Verification items for the finished model (mm, model axes). Face numbers are marked on the shaded views. A direction names the side the tool comes from. Round coordinates to 2 decimals unless told otherwise and drop trailing zeros. Order: outer loops, then holes, each group sorted by start corner. A loop starts at its lowest first (then second) coordinate and runs counter-clockwise, first axis right, second up. Notation, with made-up numbers: M 88.5,53 L 93.5,53 A33 ccw 93.5,84 Z; hole C -37.75,-11.75 d3. An arc over 180 degrees is marked long. Use one line per item in the form item = value. Start each with the question number.
Item 1: Tool access check on the marked faces 1 and 2. Record the directions out of +Z, -Z, +X, -X, +Y, -Y that give a thin tool (end or side, any length) a straight path to the whole face; none if there is none.
Item 2: Thickness scan on probe 1 along Z at (x, y) = (6, -30); probe 2 along Y at (x, z) = (9.5, 28.5); probe 3 along Y at (x, z) = (11.5, 51). Record the ranges inside material, lowest first. Write a range as [from, to].
Item 3: Go/stop test with flat-tipped pins: pin 1 Ø10 at (x, z) = (23, 29.5) entering from -Y; pin 2 Ø10 at (x, z) = (-20.5, 25) entering from +Y; pin 3 Ø5 at (x, z) = (-24, 16.5) entering from +Y. Record where each tip stops, or that it passes through.
Item 4: Cross-section at B-B on y = -24. Enter the section's corners in (x, z).
Item 5: Cross-section at A-A on y = 26.5. Count the separate pieces of the cut face and the enclosed holes in it, then the cut area to 3 significant figures.
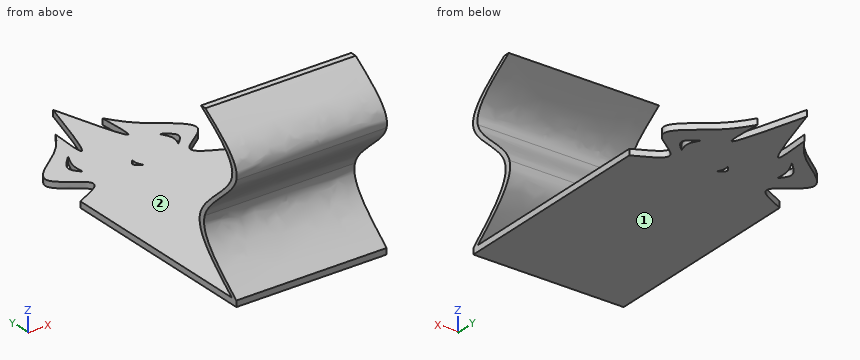
from build123d import *

# Parameters (mm, degrees)
F1_DEPTH = 2.54
F3_DEPTH = 63.5


with BuildPart() as f1:
    # F0 (on Top) → F1 (new body)
    with BuildSketch(Plane.XY):
        with BuildLine():
            Line((-31.75, -83.6839513757), (31.75, -83.6839513778))
            Line((31.75, -83.6839513778), (31.75, 5.2160486222))
            add(Edge.make_bspline(
                [(31.75, 5.2160486243), (25.7086750977, 8.2095040737), (13.2919018227, 13.2612920956), (40.4686708732, 24.151033206), (17.1693446816, 37.3717586227), (12.2441961548, 45.1813499568), (9.8845292789, 48.7718827984)],
                knots=[0, 0, 0, 0, 0.2366640156, 0.4851512444, 0.756842013, 1, 1, 1, 1], degree=3))
            add(Edge.make_bspline(
                [(9.8845292789, 48.7718827984), (10.3444855628, 41.5162894514), (11.4748144078, 23.6858829352), (4.2718916672, 48.7681543781), (0, 63.6438973943)],
                knots=[0, 0, 0, 0, 0.4069224168, 1, 1, 1, 1], degree=3))
            add(Edge.make_bspline(
                [(-9.8845292789, 48.7718827984), (-10.3444855628, 41.5162894514), (-11.4748144078, 23.6858829352), (-4.2718916672, 48.7681543781), (0, 63.6438973943)],
                knots=[0, 0, 0, 0, 0.4069224168, 1, 1, 1, 1], degree=3))
            add(Edge.make_bspline(
                [(-31.75, 5.2160486243), (-25.7086750977, 8.2095040737), (-13.2919018227, 13.2612920956), (-40.4686708732, 24.151033206), (-17.1693446816, 37.3717586227), (-12.2441961548, 45.1813499568), (-9.8845292789, 48.7718827984)],
                knots=[0, 0, 0, 0, 0.2366640156, 0.4851512444, 0.756842013, 1, 1, 1, 1], degree=3))
            Line((-31.75, 5.2160486243), (-31.75, -83.6839513757))
        make_face()
        with BuildLine():
            add(Edge.make_bspline(
                [(0, 18.4377846975), (-0.8402767268, 17.5937250168), (-2.6308980883, 15.7950420042), (-0.1427417595, 14.228570259), (1.1778091829, 13.3971894932)],
                knots=[0, 0, 0, 0, 0.4692654392, 1, 1, 1, 1], degree=3))
            add(Edge.make_bspline(
                [(0, 18.4377846975), (-0.0824907332, 17.6625700732), (-0.2575054179, 16.0178521281), (0.6814285359, 14.3035037553), (1.1778091829, 13.3971894932)],
                knots=[0, 0, 0, 0, 0.471335989, 1, 1, 1, 1], degree=3))
        make_face(mode=Mode.SUBTRACT)
        with BuildLine():
            add(Edge.make_bspline(
                [(-15.9456048132, 33.5736688751), (-16.9306722249, 31.6219338837), (-18.8522437067, 27.8146830449), (-18.5188141617, 23.8680684012), (-18.3563127499, 21.9446315956)],
                knots=[0, 0, 0, 0, 0.5126363558, 1, 1, 1, 1], degree=3))
            add(Edge.make_bspline(
                [(-18.3563127499, 21.9446315956), (-19.7054262057, 23.386298555), (-22.7926148104, 26.6852777417), (-18.411919139, 31.0924491189), (-15.9456048132, 33.5736688751)],
                knots=[0, 0, 0, 0, 0.4370039013, 1, 1, 1, 1], degree=3))
        make_face(mode=Mode.SUBTRACT)
        with BuildLine():
            add(Edge.make_bspline(
                [(18.4678306852, 28.4819673923), (19.427421291, 26.8806889301), (21.1201724035, 24.0559786368), (20.4629903584, 20.881000871), (19.9780060806, 19.4686195152), (19.7560574985, 18.8222556485)],
                knots=[0, 0, 0, 0, 0.4151573771, 0.7323521239, 1, 1, 1, 1], degree=3))
            add(Edge.make_bspline(
                [(18.4678306852, 28.4819673923), (20.8235774768, 26.9635696387), (25.4215767631, 23.9999267161), (21.6132297579, 20.51951007), (19.7560574985, 18.8222556485)],
                knots=[0, 0, 0, 0, 0.5123416723, 1, 1, 1, 1], degree=3))
        make_face(mode=Mode.SUBTRACT)
    extrude(amount=F1_DEPTH)

    # F2 (on face) → F3 (join)
    with BuildSketch(Plane.YZ.offset(31.75)):
        with BuildLine():
            add(Edge.make_bspline(
                [(-65.6484358175, 27.4432951095), (-67.9772508721, 34.9822299474), (-81.8557368461, 41.970962749), (-83.6839513778, 48.8775275409)],
                knots=[0.3464011194, 0.3464011194, 0.3464011194, 0.3464011194, 0.6770339361, 0.6770339361, 0.6770339361, 0.6770339361], degree=3))
            Line((-65.6484358175, 27.4432951095), (-63.1084358175, 27.4432951095))
            add(Edge.make_bspline(
                [(-81.1439513778, 48.8775275409), (-79.3157352707, 41.9709626757), (-65.4372513089, 34.9822301927), (-63.1084358175, 27.4432951095)],
                knots=[0.3229660639, 0.3229660639, 0.3229660639, 0.3229660639, 0.6535988806, 0.6535988806, 0.6535988806, 0.6535988806], degree=3))
            Line((-81.1439513778, 48.8775275409), (-83.6839513778, 48.8775275409))
        make_face()
        with BuildLine():
            add(Edge.make_bspline(
                [(-83.6839513778, 48.8775275409), (-85.4697730551, 55.6239420932), (-75.7576902273, 62.2919550981), (-66.0456140927, 68.9599682055)],
                knots=[0.6770339361, 0.6770339361, 0.6770339361, 0.6770339361, 1, 1, 1, 1], degree=3))
            Line((-83.6839513778, 48.8775275409), (-81.1439513778, 48.8775275409))
            add(Edge.make_bspline(
                [(-63.5056140927, 68.9599682055), (-73.2176967282, 62.2919556151), (-82.929774594, 55.6239421648), (-81.1439513778, 48.8775275409)],
                knots=[0, 0, 0, 0, 0.3229660639, 0.3229660639, 0.3229660639, 0.3229660639], degree=3))
            Line((-63.5056140927, 68.9599682055), (-66.0456140927, 68.9599682055))
        make_face()
        with BuildLine():
            add(Edge.make_bspline(
                [(-83.6839513778, 2.54), (-73.4462547351, 11.0424093805), (-63.2085565888, 19.5448188091), (-65.6484358175, 27.4432951095)],
                knots=[0, 0, 0, 0, 0.3464011194, 0.3464011194, 0.3464011194, 0.3464011194], degree=3))
            Line((-83.6839513778, 2.54), (-81.1439513778, 2.54))
            add(Edge.make_bspline(
                [(-63.1084358175, 27.4432951095), (-60.6685561312, 19.5448185522), (-70.9062511318, 11.0424082477), (-81.1439513778, 2.54)],
                knots=[0.6535988806, 0.6535988806, 0.6535988806, 0.6535988806, 1, 1, 1, 1], degree=3))
            Line((-63.1084358175, 27.4432951095), (-65.6484358175, 27.4432951095))
        make_face()
    extrude(amount=-F3_DEPTH)


solid = f1.part
Output values:
q1.face_1 = -Z, +X, -X, +Y, -Y
q1.face_2 = +X, -X, +Y
q2.probe_1 = [0, 2.54]
q2.probe_2 = [-66.05, -63.51]
q2.probe_3 = [-83.88, -81.34]
q3.pin_1 = -70.63
q3.pin_2 = -62.74
q3.pin_3 = -64.63
q4.outline = M -31.75,0 L 31.75,0 L 31.75,2.54 L -31.75,2.54 Z
q5.separate_pieces = 3
q5.enclosed_holes = 0
q5.area = 149 mm2
